Design review of the part built by this model. Coordinates are the model's own, in mm. A direction names the side the tool comes from. Give positions to 0.01 mm unless a question says otherwise; leave off trailing zeros. Loops run counter-clockwise (first coordinate to the right, second up) from the corner with the lowest first, then second, coordinate; pieces in that order, holes last. Notation, with made-up numbers: (-12, 24) -> (44, 24) arc R30 ccw to (44, 52) -> close; hole circle Ø9 at (-29, 87.25). An arc over 180 degrees is marked (long way). Answer in a Markdown table with one row per item. Add a question column.
(1) Consider section C-C on y = -71.5. Write out the cut boundary in (x, z) (3 decimals).
(2) Draft analysis for pull direction Z (two halves, no side actions). For faces 4 (the cylindrical face through (0, 0, 6)), 5 (the cylindrical face through (0.089, 38.748, -123.043)), 6 (the flat face through (7.5, 6, 2)), state which applies: +Z half, -Z half, draft (parallel to the pull), parting line (faces both ways), or undercut.
(3) Consider section D-D on z = -56. Write out the cut boundary in (x, y) (3 decimals), then the cut area to 3 significant figures.
(4) For line 1 (Y direction, x = -3.75, z = 0); line 2 (Z direction, x = 0.25, y = 40.5); line 3 (Z direction, x = 4, y = 72), list the stretches that pass through material, from the lowest coordinate up.
(5) For pin 1 (20 mm diameter, centred on y = -50, z = -2, fed in from +X); pin 2 (14.5 mm diameter, centred on y = -55.5, z = -3.5, fed in from -X); pin 3 (1.5 mm diameter, centred on x = 0.5, z = -40, fed in from +Y); pin 4 (9.5 mm diameter, centred on y = 0, z = 0, fed in from -X), all flat-tipped, find the tip position at first contact; note any pin that passes through.
(6) Consider section A-A on z = 0. Write out the cut boundary in (x, y) (3 decimals), then the cut area to 3 significant figures.
(7) For faces 1 (the cylindrical face through (0.1, 5.4, 5.9)), 2 (the flat face through (-0.5, 0, 80)), 3 (the flat face through (0.5, 0, 80)), list the 3-axis set-ups (+Z, -Z, +X, -X, +Y, -Y) from which the entire face can be reached by the end or side of a thin tool; tool diameter is ignored.
from build123d import *

# Parameters (mm, degrees)
SKETCH1_R           = 129
SKETCH1_R_2         = 125
BOSS_EXTRUDE1_DEPTH = 6.375
BOSS_EXTRUDE2_DEPTH = 0.5
SKETCH2_4_R         = 8
SKETCH2_4_R_2       = 6
BOSS_EXTRUDE3_DEPTH = 7.5


with BuildPart() as part:
    # Sketch1 → Boss-Extrude1 (new, symmetric)
    with BuildSketch(Plane(origin=(0, 0, 0), x_dir=(0, 0, -1), z_dir=(1, 0, 0))):
        Circle(SKETCH1_R)
        Circle(SKETCH1_R_2, mode=Mode.SUBTRACT)
    extrude(amount=BOSS_EXTRUDE1_DEPTH, both=True)

    # Sketch2 → Boss-Extrude2 (add, symmetric)
    with BuildSketch(Plane(origin=(0, 0, 0), x_dir=(0, 0, -1), z_dir=(1, 0, 0))):
        with BuildLine():
            ThreePointArc((-3.768738548, 7.056671294), (0.113394951, 7.999196309), (3.9672518, 6.947007496))
            Line((3.9672518, 6.947007496), (9.107052817, 124.667804942))
            ThreePointArc((9.107052817, 124.667804942), (0.101595075, 124.999958714), (-8.904390692, 124.682443938))
            Line((-8.904390692, 124.682443938), (-3.768738548, 7.056671294))
        make_face()
        with BuildLine():
            ThreePointArc((-7.056671294, -3.768738548), (-7.999196309, 0.113394951), (-6.947007496, 3.9672518))
            Line((-6.947007496, 3.9672518), (-124.667804942, 9.107052817))
            ThreePointArc((-124.667804942, 9.107052817), (-124.999958714, 0.101595075), (-124.682443938, -8.904390692))
            Line((-124.682443938, -8.904390692), (-7.056671294, -3.768738548))
        make_face()
        with BuildLine():
            Line((124.682443938, 8.904390692), (7.056671294, 3.768738548))
            ThreePointArc((7.056671294, 3.768738548), (7.760585363, 1.942502207), (8, 0))
            ThreePointArc((8, 0), (7.732271981, -2.05230846), (6.947007496, -3.9672518))
            Line((6.947007496, -3.9672518), (124.667804942, -9.107052817))
            ThreePointArc((124.667804942, -9.107052817), (124.916923629, -4.556554745), (125, 0))
            ThreePointArc((125, 0), (124.920585758, 4.455025686), (124.682443938, 8.904390692))
        make_face()
        with BuildLine():
            Line((8.904390692, -124.682443938), (3.768738548, -7.056671294))
            ThreePointArc((3.768738548, -7.056671294), (-0.113394951, -7.999196309), (-3.9672518, -6.947007496))
            Line((-3.9672518, -6.947007496), (-9.107052817, -124.667804942))
            ThreePointArc((-9.107052817, -124.667804942), (-0.101595075, -124.999958714), (8.904390692, -124.682443938))
        make_face()
    extrude(amount=BOSS_EXTRUDE2_DEPTH, both=True)

    # Sketch2_4 → Boss-Extrude3 (add, symmetric)
    with BuildSketch(Plane(origin=(0, 0, 0), x_dir=(0, 0, -1), z_dir=(1, 0, 0))):
        Circle(SKETCH2_4_R)
        Circle(SKETCH2_4_R_2, mode=Mode.SUBTRACT)
    extrude(amount=BOSS_EXTRUDE3_DEPTH, both=True)


solid = part.part
Values follow:
| question | item | result |
|---|---|---|
| 1 | outline | (-6.375, -107.372) -> (6.375, -107.372) -> (6.375, -102.532) -> (-6.375, -102.532) -> close; (-6.375, 102.532) -> (6.375, 102.532) -> (6.375, 107.372) -> (-6.375, 107.372) -> close; (-0.5, -6.582) -> (0.5, -6.582) -> (0.5, 6.786) -> (-0.5, 6.786) -> close |
| 2 | face 4 | undercut |
| 2 | face 5 | parting line |
| 2 | face 6 | draft |
| 3 | outline | (-6.375, -116.211) -> (6.375, -116.211) -> (6.375, -111.754) -> (-6.375, -111.754) -> close; (-6.375, 111.754) -> (6.375, 111.754) -> (6.375, 116.211) -> (-6.375, 116.211) -> close; (-0.5, -6.109) -> (0.5, -6.109) -> (0.5, 5.906) -> (-0.5, 5.906) -> close |
| 3 | area | 126 mm2 |
| 4 | line 1 | -129 to -125, -8 to -6, 6 to 8, 125 to 129 |
| 4 | line 2 | -122.48 to -118.26, -5.43 to 5.23, 118.26 to 122.48 |
| 4 | line 3 | -107.04 to -102.18, 102.18 to 107.04 |
| 5 | pin 1 | x = 0.5 |
| 5 | pin 2 | x = -0.5 |
| 5 | pin 3 | y = 122.88 |
| 5 | pin 4 | through |
| 6 | outline | (-7.5, -8) -> (-0.5, -8) -> (-0.5, -125) -> (-6.375, -125) -> (-6.375, -129) -> (6.375, -129) -> (6.375, -125) -> (0.5, -125) -> (0.5, -8) -> (7.5, -8) -> (7.5, -6) -> (-7.5, -6) -> close; (-7.5, 6) -> (7.5, 6) -> (7.5, 8) -> (0.5, 8) -> (0.5, 125) -> (6.375, 125) -> (6.375, 129) -> (-6.375, 129) -> (-6.375, 125) -> (-0.5, 125) -> (-0.5, 8) -> (-7.5, 8) -> close |
| 6 | area | 396 mm2 |
| 7 | face 1 | none |
| 7 | face 2 | -X |
| 7 | face 3 | +X |
